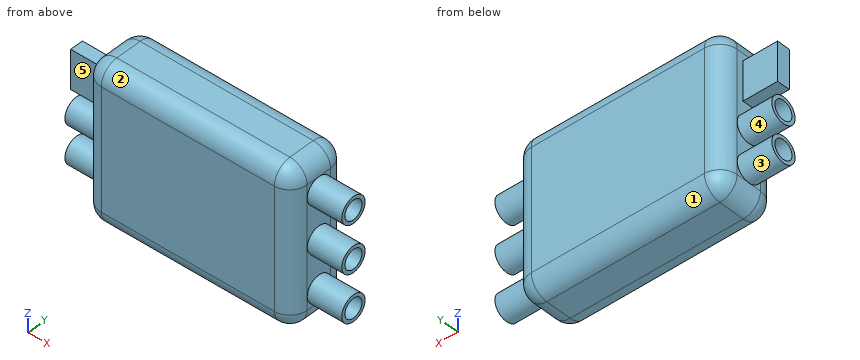
```python
from build123d import *

# Parameters (mm, degrees)
BOSS_EXTRUDE1_DEPTH = 7
FILLET1_R           = 2
SKETCH2_R           = 1.5
SKETCH2_R_2         = 1.1
BOSS_EXTRUDE2_DEPTH = 4
SKETCH3_R           = 1.5
SKETCH3_R_2         = 1.1
SKETCH3_W           = 4.5
SKETCH3_H           = 1.5
BOSS_EXTRUDE3_DEPTH = 4


with BuildPart() as part:
    # Sketch1 → Boss-Extrude1 (new body)
    with BuildSketch(Plane(origin=(0, 0, 0), x_dir=(1, 0, 0), z_dir=(0, 1, 0))):
        with BuildLine():
            Line((-10, 9), (10, 9))
            ThreePointArc((10, 9), (11.414213562, 8.414213562), (12, 7))
            Line((12, 7), (12, -7))
            ThreePointArc((12, -7), (11.414213562, -8.414213562), (10, -9))
            Line((10, -9), (-10, -9))
            ThreePointArc((-10, -9), (-11.414213562, -8.414213562), (-12, -7))
            Line((-12, -7), (-12, 7))
            ThreePointArc((-12, 7), (-11.414213562, 8.414213562), (-10, 9))
        make_face()
    extrude(amount=BOSS_EXTRUDE1_DEPTH)

    # Fillet1
    fillet1_edges = [part.edges().sort_by_distance(p)[0] for p in [
        (12, 0, 0),
        (11.414213562, 0, 8.414213562),
        (0, 0, 9),
        (-11.414213562, 0, 8.414213562),
        (11.414213562, 7, 8.414213562),
        (12, 7, 0),
        (11.414213562, 7, -8.414213562),
        (0, 7, -9),
        (-11.414213562, 7, -8.414213562),
        (-12, 7, 0),
        (-11.414213562, 7, 8.414213562),
        (-12, 0, 0),
        (0, 7, 9),
        (-11.414213562, 0, -8.414213562),
        (0, 0, -9),
        (11.414213562, 0, -8.414213562),
    ]]
    fillet(fillet1_edges, radius=FILLET1_R)

    # Sketch2 → Boss-Extrude2 (add)
    # profile 1 of 3: a face of its own
    with BuildSketch(Plane(origin=(12, 0, 0), x_dir=(0, 0, -1), z_dir=(1, 0, 0))):
        with Locations(Location((0, 3.5, 0), (0, 0, 270))):
            Circle(SKETCH2_R)
        with Locations((0, 3.5)):
            Circle(SKETCH2_R_2, mode=Mode.SUBTRACT)
    # profile 2 of 3: a face of its own
    with BuildSketch(Plane(origin=(12, 0, 0), x_dir=(0, 0, -1), z_dir=(1, 0, 0))):
        with Locations(Location((-5.5, 3.5, 0), (0, 0, 180))):
            Circle(SKETCH2_R)
        with Locations((-5.5, 3.5)):
            Circle(SKETCH2_R_2, mode=Mode.SUBTRACT)
    # profile 3 of 3: a face of its own
    with BuildSketch(Plane(origin=(12, 0, 0), x_dir=(0, 0, -1), z_dir=(1, 0, 0))):
        with Locations(Location((5.479960671, 3.5, 0), (0, 0, 270))):
            Circle(SKETCH2_R)
        with Locations((5.479960671, 3.5)):
            Circle(SKETCH2_R_2, mode=Mode.SUBTRACT)
    extrude(amount=BOSS_EXTRUDE2_DEPTH)

    # Sketch3 → Boss-Extrude3 (add)
    # profile 1 of 3: a face of its own
    with BuildSketch(Plane.ZY.offset(12)):
        with Locations(Location((-5.5, 3.5, 0), (0, 0, 180))):
            Circle(SKETCH3_R)
        with Locations((-5.5, 3.5)):
            Circle(SKETCH3_R_2, mode=Mode.SUBTRACT)
    # profile 2 of 3: a face of its own
    with BuildSketch(Plane.ZY.offset(12)):
        with Locations(Location((-1.1, 3.5, 0), (0, 0, 270))):
            Circle(SKETCH3_R)
        with Locations((-1.1, 3.5)):
            Circle(SKETCH3_R_2, mode=Mode.SUBTRACT)
    # profile 3 of 3: a face of its own
    with BuildSketch(Plane.ZY.offset(12)):
        with Locations((3.921006342, 3.5)):
            Rectangle(SKETCH3_W, SKETCH3_H)
    extrude(amount=BOSS_EXTRUDE3_DEPTH)


solid = part.part
```
Geometry check sheet. Reference: the model listing, model coordinates, mm. Face numbers are marked on the shaded views. A direction names the side the tool comes from. Give positions to 0.01 mm unless a question says otherwise; leave off trailing zeros. Write each loop counter-clockwise with the first axis right and the second up, starting at its lowest first coordinate (ties: lowest second). Pieces come first, ordered by that corner, then holes. Notation, with made-up numbers: (87, 52) - (95, 52) arc R11 ccw to (95, 59) - close; hole circle Ø6 at (67, 47). An arc over 180 degrees is marked (long way). Use a Markdown table: item, result.
Q1. Thickness scan on L1, parallel to Y at x = -13.65, z = -5.5; L2, parallel to X at y = 3, z = 1.75; L3, parallel to X at y = 4.5, z = -4. Record the ranges inside material, lowest first. Write a range as [from, to].
Computed:
| item | result |
|---|---|
| L1 | y = [2, 2.4], [4.6, 5] |
| L2 | x = [-16, 12] |
| L3 | x = [-12, 12] |
Q2. Section check C-C, the plane y = 0.5. Enter the section's corners in (x, z).
Computed:
| item | result |
|---|---|
| outline | (-11.32, -7) arc R1.32 ccw to (-10, -8.32) - (10, -8.32) arc R1.32 ccw to (11.32, -7) - (11.32, 7) arc R1.32 ccw to (10, 8.32) - (-10, 8.32) arc R1.32 ccw to (-11.32, 7) - close |
Q3. Set-up check for the marked faces 4 and 5: record each of +Z, -Z, +X, -X, +Y, -Y from which the full face is reachable in a straight line by a thin tool's end or side.
Computed:
| item | result |
|---|---|
| face 4 | -X |
| face 5 | +Z, -X, -Y |
Q4. Section check B-B, the plane x = 1. Enter the section's corners in (y, z), then the cut area to 3 significant figures.
Computed:
| item | result |
|---|---|
| outline | (0, -7) arc R2 ccw to (2, -9) - (5, -9) arc R2 ccw to (7, -7) - (7, 7) arc R2 ccw to (5, 9) - (2, 9) arc R2 ccw to (0, 7) - close |
| area | 123 mm² |
Q5. Draft check along Z on the marked faces 1, 2 and 3. Enter one of: pulls with the +Z half, pulls with the -Z half, needs draft (parallel to the pull), parting line crosses it, or undercut.
Computed:
| item | result |
|---|---|
| face 1 | pulls with the -Z half |
| face 2 | pulls with the +Z half |
| face 3 | undercut |
Q6. Section check A-A, the plane x = 12.5. Enter the section's corners in (y, z).
Computed:
| item | result |
|---|---|
| outline | circle Ø3 at (3.5, -5.48); circle Ø3 at (3.5, 0); circle Ø3 at (3.5, 5.5); hole circle Ø2.2 at (3.5, -5.48); hole circle Ø2.2 at (3.5, 0); hole circle Ø2.2 at (3.5, 5.5) |
Q7. Go/stop test with flat-tipped pins: P1, Ø1.6, axis at x = -14, y = 4, coming from the +Z side; P2, Ø4, axis at x = -6, y = 5.5, coming from the -Z side; P3, Ø3, axis at x = -13, z = 3.5, coming from the +Y side; P4, Ø2, axis at y = 1, z = 5, coming from the -X side. Record where each tip stops, or that it passes through.
Computed:
| item | result |
|---|---|
| P1 | stops at z = 6.17 |
| P2 | stops at z = -9 |
| P3 | stops at y = 6.32 |
| P4 | stops at x = -12 |
